Geometry: final body of the model. Coordinates: model frame, mm. A direction names the side the tool comes from. Coordinates: 2 decimals unless noted, no trailing zeros. Write each loop counter-clockwise with the first axis right and the second up, starting at its lowest first coordinate (ties: lowest second). Pieces come first, ordered by that corner, then holes. Notation, with made-up numbers: M 6,48.25 L 22,48.25 A18 cw 22,60.25 Z; hole C -31,-31.75 d2. An arc over 180 degrees is marked long. Write item = value, one per line. Start each with the question number.
Item 1: Section A-A on x = -5. Output: boundary loops of the cut face in (y, z).
Item 2: Pull-direction query (X, two-part tool) for faces 4 (the cylindrical face through (-0.54, 14.11, 12.69)), 5 (the flat face through (12, 25.119, 5)); classes: +X half, -X half, draft (parallel to the pull), parting line (faces both ways), or undercut.
Item 3: First-contact query: pin 1 Ø2 at (x, y) = (-10, 7.5) entering from -Z; pin 2 Ø2 at (y, z) = (14, -15.5) entering from -X; pin 3 Ø1 at (y, z) = (12, -9) entering from +X; pin 4 Ø5 at (y, z) = (15.5, -14) entering from +X. Flat tips, straight axial feed; report the tip coordinate or a pass-through.
Item 4: Ray query, L1, parallel to X at y = 18, z = 0; L2, parallel to Y at x = -15.5, z = -1; L3, parallel to Z at x = 0, y = 8.5. Return the intervals inside material, ascending. Write a range as [from, to].
Item 5: Section B-B on z = -6. Output: boundary loops of the cut face in (x, y).
Item 6: Section C-C on x = 0. Output: boundary loops of the cut face in (y, z).
Item 7: Reachability of faces 1 (the flat face through (-6.4, 2.789, 11.4)), 2 (the flat face through (6, 4.239, -13)), 3 (the flat face through (-1, 11.6, -13.9)) from +Z, -Z, +X, -X, +Y, -Y: full face, straight path, thin tool, end or side. Return the list, or none.
Item 8: Section D-D on y = 20.75. Output: boundary loops of the cut face in (x, z).
from build123d import *

# Parameters (mm, degrees)
SKETCH2_W          = 2
SKETCH2_H          = 66.093473653
CUT_EXTRUDE1_DEPTH = 23.33


with BuildPart() as part:
    # Sketch1 → Revolve1 (revolve)
    with BuildSketch(Plane.XY):
        Polygon((12.7, 2.789418738), (12.7, 25.119418738), (14.15, 25.119418738), (14.15, 4.239418738), (17.15, 4.239418738), (17.15, 2.789418738), align=None)
    revolve(axis=Axis((0, 0, 0), (0, 1, 0)))

    # Sketch2 → Cut-Extrude1 (cut, through all)
    with BuildSketch(Plane(origin=(0, 25.119418738, 0), x_dir=(1, 0, 0), z_dir=(0, 1, 0))):
        with Locations((0, 26.994107081)):
            Rectangle(SKETCH2_W, SKETCH2_H)
    extrude(amount=-CUT_EXTRUDE1_DEPTH, mode=Mode.SUBTRACT)


solid = part.part
Responses:
q1.outline = M 2.79,-16.4 L 4.24,-16.4 L 4.24,-13.24 L 25.12,-13.24 L 25.12,-11.67 L 2.79,-11.67 Z; M 2.79,11.67 L 25.12,11.67 L 25.12,13.24 L 4.24,13.24 L 4.24,16.4 L 2.79,16.4 Z
q2.face_4 = undercut
q2.face_5 = draft
q3.pin_1 = -10.92
q3.pin_2 = through
q3.pin_3 = 11.31
q3.pin_4 = 8.24
q4.L1 = [-14.15, -12.7], [12.7, 14.15]
q4.L2 = [2.79, 4.24]
q4.L3 = [12.7, 14.15]
q5.outline = M -16.07,2.79 L -11.19,2.79 L -11.19,25.12 L -12.81,25.12 L -12.81,4.24 L -16.07,4.24 Z; M 11.19,2.79 L 16.07,2.79 L 16.07,4.24 L 12.81,4.24 L 12.81,25.12 L 11.19,25.12 Z
q6.outline = M 2.79,12.7 L 25.12,12.7 L 25.12,14.15 L 4.24,14.15 L 4.24,17.15 L 2.79,17.15 Z
q7.face_1 = +Z, -Z, +X, -X, -Y
q7.face_2 = +Y
q7.face_3 = -Z, +Y, -Y
q8.outline = M -1,-14.11 L -1,-12.66 A12.7 cw long 1,-12.66 L 1,-14.11 A14.15 ccw long Z
